from build123d import *

# Parameters (mm, degrees)
CROQUIS3_W              = 16
CROQUIS3_H              = 39.75
SALIENTE_EXTRUIR1_DEPTH = 1.6
CROQUIS4_W              = 5
CROQUIS4_H              = 5.5
CROQUIS4_W_2            = 5.3
CROQUIS4_H_2            = 5.3
SALIENTE_EXTRUIR2_DEPTH = 1
CROQUIS5_W              = 6.792082101
CROQUIS5_H              = 13.5
SALIENTE_EXTRUIR3_DEPTH = 6
CROQUIS6_W              = 3.207917899
CROQUIS6_H              = 11
SALIENTE_EXTRUIR4_DEPTH = 3.5
CROQUIS7_W              = 8
CROQUIS7_H              = 3
SALIENTE_EXTRUIR5_DEPTH = 2.5
SALIENTE_EXTRUIR6_DEPTH = 3
CROQUIS9_R              = 1.5
CORTAR_EXTRUIR1_DEPTH   = 23.248946604
SALIENTE_EXTRUIR7_DEPTH = 2
CROQUIS11_W             = 7
CROQUIS11_H             = 4
CROQUIS11_W_2           = 4
CROQUIS11_H_2           = 12
SALIENTE_EXTRUIR8_DEPTH = 1.5


with BuildPart() as part:
    # Croquis3 → Saliente-Extruir1 (new body)
    with BuildSketch(Plane.XY):
        Rectangle(CROQUIS3_W, CROQUIS3_H)
    extrude(amount=SALIENTE_EXTRUIR1_DEPTH)

    # Croquis4 → Saliente-Extruir2 (add)
    with BuildSketch(Plane.XY.offset(1.6)):
        with Locations((0, 3.625)):
            Rectangle(CROQUIS4_W, CROQUIS4_H)
        with Locations((-1.15, -16.575)):
            Rectangle(CROQUIS4_W_2, CROQUIS4_H_2)
    extrude(amount=SALIENTE_EXTRUIR2_DEPTH)

    # Croquis5 → Saliente-Extruir3 (add)
    with BuildSketch(Plane.XY.offset(1.6)):
        with Locations((4.603958949, -6.625)):
            Rectangle(CROQUIS5_W, CROQUIS5_H)
    extrude(amount=SALIENTE_EXTRUIR3_DEPTH)

    # Croquis6 → Saliente-Extruir4 (add)
    with BuildSketch(Plane.XY.offset(1.6)):
        with Locations((-0.39604105, -6.625)):
            Rectangle(CROQUIS6_W, CROQUIS6_H)
    extrude(amount=SALIENTE_EXTRUIR4_DEPTH)

    # Croquis7 → Saliente-Extruir5 (add)
    with BuildSketch(Plane.XY.offset(1.6)):
        with Locations((0.5, 8.875)):
            Rectangle(CROQUIS7_W, CROQUIS7_H)
    extrude(amount=SALIENTE_EXTRUIR5_DEPTH)

    # Croquis8 → Saliente-Extruir6 (add, symmetric)
    with BuildSketch(Plane.ZY.offset(-0.5)):
        Polygon((4.1, 9.375), (4.6, 9.375), (4.6, 16.375), (5.6, 16.375), (5.6, 8.375), (4.1, 8.375), align=None)
    extrude(amount=SALIENTE_EXTRUIR6_DEPTH, both=True)

    # Croquis9 → Cortar-Extruir1 (cut, through all)
    with BuildSketch(Plane.XY.offset(1.6)):
        with Locations((5.55, 17.525)):
            Circle(CROQUIS9_R)
        with Locations((-5.35, 17.525)):
            Circle(CROQUIS9_R)
        with Locations((5.55, 3.025)):
            Circle(CROQUIS9_R)
        with Locations((5.55, -15.925)):
            Circle(CROQUIS9_R)
    extrude(amount=-CORTAR_EXTRUIR1_DEPTH, mode=Mode.SUBTRACT)

    # Croquis10 → Saliente-Extruir7 (add, symmetric)
    with BuildSketch(Plane(origin=(8, -13.375, 4.6), x_dir=(-1, 0, 0), z_dir=(0, 0, -1))):
        Polygon((0, 12.75), (-1.6, -0.814858061), (-1.302065369, -0.85), (0, 10.188957451), align=None)
    extrude(amount=SALIENTE_EXTRUIR7_DEPTH, both=True)

    # Croquis11 → Saliente-Extruir8 (add)
    with BuildSketch(Plane(origin=(0, 0, 0), x_dir=(-1, 0, 0), z_dir=(0, 0, -1))):
        with Locations((0, 8.875)):
            Rectangle(CROQUIS11_W, CROQUIS11_H)
        with Locations((1, -6.625)):
            Rectangle(CROQUIS11_W_2, CROQUIS11_H_2)
    extrude(amount=SALIENTE_EXTRUIR8_DEPTH)


solid = part.part
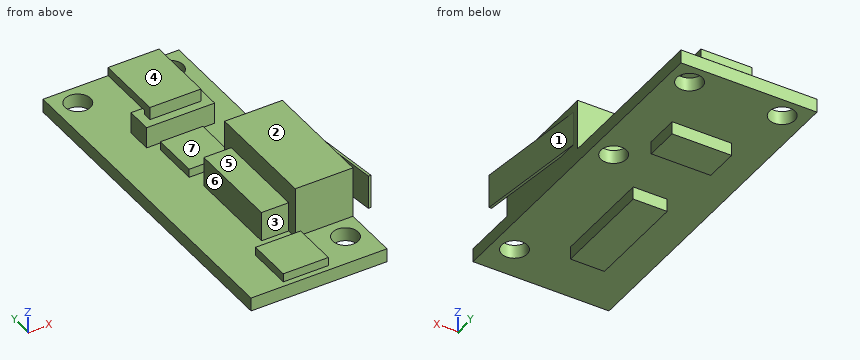
Verification items for the finished model (mm, model axes). Face numbers are marked on the shaded views. A direction names the side the tool comes from. Coordinates: 2 decimals unless noted, no trailing zeros. Loops run counter-clockwise (first coordinate to the right, second up) from the corner with the lowest first, then second, coordinate; pieces in that order, holes last. Notation, with made-up numbers: (-37, 60.5) -> (-1, 60.5) arc R6 ccw to (-1, 67.5) -> close; hole circle Ø3 at (85.25, 64.25). An arc over 180 degrees is marked (long way). Answer as a JSON object with one key per item and string values. Group by question number.
Item 1: Sectioned sample at B-B on x = 5.55. Record the boundary of the cut face in (y, z) (3 decimals), plus the area to 3 significant figures.
Item 2: Sectioned sample at D-D on z = 0.5. Record the boundary of the cut face in (x, y) (3 decimals).
Item 3: Tool access check on the marked faces 4, 5, 6 and 7. Record the directions out of +Z, -Z, +X, -X, +Y, -Y that give a thin tool (end or side, any length) a straight path to the whole face; none if there is none.
Item 4: Depth check by flat-ended pin: pin 1 (1.6 mm diameter, centred on y = 9, z = -0.5, fed in from +X); pin 2 (0.8 mm diameter, centred on x = 0.5, z = 4.5, fed in from -Y) (3 decimals); pin 3 (3 mm diameter, centred on x = 4, z = 4, fed in from -Y) (3 decimals). Enter the tip coordinate at first touch or a pass-through.
Item 5: Scan lines: probe 1 along Y at (x, z) = (5.55, 1.3) (3 decimals); probe 2 along Y at (x, z) = (-5.35, 0.4) (3 decimals); probe 3 along Y at (x, z) = (6.25, 0.5) (3 decimals). Record each from-to range of solid material in increasing order.
Item 6: Sectioned sample at A-A on y = 12.5. Record the boundary of the cut face in (x, z), plus the area to 3 significant figures.
Item 7: Mould release check, pull along Y, two halves, no side actions. Record for the marked faces 1, 2 and 3: +Y half, -Y half, draft (parallel to the pull), parting line (faces both ways), or undercut.
Item 8: Sectioned sample at C-C on x = -5.35. Record the boundary of the cut face in (y, z) (3 decimals).
Evaluation:
{
 "1": {"outline": "(-19.875, 0) -> (-17.425, 0) -> (-17.425, 1.6) -> (-19.875, 1.6) -> close; (-14.425, 0) -> (1.525, 0) -> (1.525, 1.6) -> (0.125, 1.6) -> (0.125, 7.6) -> (-13.375, 7.6) -> (-13.375, 1.6) -> (-14.425, 1.6) -> close; (4.525, 0) -> (16.025, 0) -> (16.025, 1.6) -> (4.525, 1.6) -> close; (19.025, 0) -> (19.875, 0) -> (19.875, 1.6) -> (19.025, 1.6) -> close", "area": "130 mm²"},
 "2": {"outline": "(-8, -19.875) -> (8, -19.875) -> (8, 19.875) -> (-8, 19.875) -> close; hole circle Ø3 at (-5.35, 17.525); hole circle Ø3 at (5.55, -15.925); hole circle Ø3 at (5.55, 3.025); hole circle Ø3 at (5.55, 17.525)"},
 "3": {"face 4": "+Z, +X, -X, +Y", "face 5": "+Z, -X, -Y", "face 6": "+Z, -X", "face 7": "+Z, +X, -X"},
 "4": {"pin 1": "stops at x = 8", "pin 2": "stops at y = -12.125", "pin 3": "stops at y = -13.375"},
 "5": {"probe 1": "y = -19.875 to -17.425, -14.425 to 1.525, 4.525 to 16.025, 19.025 to 19.875", "probe 2": "y = -19.875 to 16.025, 19.025 to 19.875", "probe 3": "y = -19.875 to -17.252, -14.598 to 1.698, 4.352 to 16.198, 18.852 to 19.875"},
 "6": {"outline": "(-8, 0) -> (8, 0) -> (8, 1.6) -> (-8, 1.6) -> close; (-2.5, 4.6) -> (3.5, 4.6) -> (3.5, 5.6) -> (-2.5, 5.6) -> close", "area": "31.6 mm²"},
 "7": {"face 1": "+Y half", "face 2": "draft", "face 3": "undercut"},
 "8": {"outline": "(-19.875, 0) -> (16.025, 0) -> (16.025, 1.6) -> (-19.875, 1.6) -> close; (19.025, 0) -> (19.875, 0) -> (19.875, 1.6) -> (19.025, 1.6) -> close"}
}
